from build123d import *

# Parameters (mm, degrees)
ESBO_O1_W                = 175
ESBO_O1_H                = 172.5
RESSALTO_EXTRUS_O1_DEPTH = 10
ESBO_O5_W                = 30
ESBO_O5_H                = 6
RESSALTO_EXTRUS_O5_DEPTH = 10
ESBO_O6_W                = 6
ESBO_O6_H                = 30
RESSALTO_EXTRUS_O6_DEPTH = 10
ESBO_O7_W                = 30
ESBO_O7_H                = 6
RESSALTO_EXTRUS_O7_DEPTH = 10
ESBO_O9_W                = 6.2
ESBO_O9_H                = 172.5
CORTE_EXTRUS_O2_DEPTH    = 5
ESBO_O10_R               = 1.5
CORTE_EXTRUS_O3_DEPTH    = 8
ESBO_O11_R               = 1.5
CORTE_EXTRUS_O4_DEPTH    = 8


with BuildPart() as part:
    # Esboço1 → Ressalto-extrusão1 (new body)
    with BuildSketch(Plane.XY):
        Rectangle(ESBO_O1_W, ESBO_O1_H)
    extrude(amount=RESSALTO_EXTRUS_O1_DEPTH)

    # Esboço5 → Ressalto-extrusão5 (add)
    with BuildSketch(Plane(origin=(0, 86.25, 0), x_dir=(1, 0, 0), z_dir=(0, 1, 0))):
        with Locations((-37.5, -5)):
            Rectangle(ESBO_O5_W, ESBO_O5_H)
        with Locations((37.5, -5)):
            Rectangle(ESBO_O5_W, ESBO_O5_H)
    extrude(amount=RESSALTO_EXTRUS_O5_DEPTH)

    # Esboço6 → Ressalto-extrusão6 (add)
    with BuildSketch(Plane.ZY.offset(87.5)):
        with Locations((5, 36.25)):
            Rectangle(ESBO_O6_W, ESBO_O6_H)
        with Locations((5, -36.25)):
            Rectangle(ESBO_O6_W, ESBO_O6_H)
    extrude(amount=RESSALTO_EXTRUS_O6_DEPTH)

    # Esboço7 → Ressalto-extrusão7 (add)
    with BuildSketch(Plane.XZ.offset(86.25)):
        with Locations((-37.5, 5)):
            Rectangle(ESBO_O7_W, ESBO_O7_H)
        with Locations((37.5, 5)):
            Rectangle(ESBO_O7_W, ESBO_O7_H)
    extrude(amount=RESSALTO_EXTRUS_O7_DEPTH)

    # Esboço9 → Corte-extrusão2 (cut)
    with BuildSketch(Plane.XY.offset(10)):
        with Locations((79.4, 0)):
            Rectangle(ESBO_O9_W, ESBO_O9_H)
    extrude(amount=-CORTE_EXTRUS_O2_DEPTH, mode=Mode.SUBTRACT)

    # Esboço10 → Corte-extrusão3 (cut)
    with BuildSketch(Plane.ZY.offset(87.5)):
        with Locations((5, -71.25)):
            Circle(ESBO_O10_R)
    extrude(amount=-CORTE_EXTRUS_O3_DEPTH, mode=Mode.SUBTRACT)

    # Esboço11 → Corte-extrusão4 (cut)
    with BuildSketch(Plane.XZ.offset(86.25)):
        with Locations((65, 5)):
            Circle(ESBO_O11_R)
    extrude(amount=-CORTE_EXTRUS_O4_DEPTH, mode=Mode.SUBTRACT)


solid = part.part
The model under review builds one solid part; all positions refer to its coordinate system, in mm. A direction names the side the tool comes from. Give positions to 0.01 mm unless a question says otherwise; leave off trailing zeros. Loops run counter-clockwise (first coordinate to the right, second up) from the corner with the lowest first, then second, coordinate; pieces in that order, holes last. Notation, with made-up numbers: (42, 19) -> (89, 19) arc R23 cw to (89, 41) -> close; hole circle Ø11 at (29.25, 5). An arc over 180 degrees is marked (long way). Write each question's results on one line, items separated by ' | '.
1) Tool access review of faces 1 (the face through (82.5, -1, 8)), 2 (the face through (37, 91, 8)), 3 (the face through (-92, -36, 2)), 4 (the face through (52.5, -91, 5)), 5 (the face through (-92, -51.25, 5)): name each direction out of +Z, -Z, +X, -X, +Y, -Y from which nothing blocks a thin tool from reaching the whole face with its end or side.
Conclusion:
face 1: +Z, +Y, -Y | face 2: +Z, +X, -X, +Y | face 3: -Z, -X, +Y, -Y | face 4: +Z, -Z, +X, -Y | face 5: +Z, -Z, -X, -Y
2) Take a section at A-A, the plane y = 73. Give the boundary of the cut face in (x, z), plus the area to 3 significant figures.
Conclusion:
outline: (-87.5, 0) -> (87.5, 0) -> (87.5, 10) -> (82.5, 10) -> (82.5, 5) -> (76.3, 5) -> (76.3, 10) -> (-87.5, 10) -> close | area: 1,720 mm^2
3) For line 1 along Z through (x, y) = (65, -81.5); line 2 along X through (y, z) = (-80.5, 7); line 3 along X through (y, z) = (-43.5, 7.25), list the stretches that pass through material, from the lowest coordinate up. Write a range as from..to.
Conclusion:
line 1: z = 0..3.5, 6.5..10 | line 2: x = -87.5..76.3, 82.5..87.5 | line 3: x = -97.5..76.3, 82.5..87.5
4) Draft analysis for pull direction X (two halves, no side actions). For faces 6 (the face through (-97.5, -36, 5)), 7 (the face through (-92, 21.25, 5)), 8 (the face through (22.5, -91, 5)), state which applies: pulls with the +X half, pulls with the -X half, needs draft (parallel to the pull), parting line crosses it, or undercut.
Conclusion:
face 6: pulls with the -X half | face 7: needs draft | face 8: undercut
5) Take a section at C-C, the plane x = 49. Give the boundary of the cut face in (y, z).
Conclusion:
outline: (-96.25, 2) -> (-86.25, 2) -> (-86.25, 0) -> (86.25, 0) -> (86.25, 2) -> (96.25, 2) -> (96.25, 8) -> (86.25, 8) -> (86.25, 10) -> (-86.25, 10) -> (-86.25, 8) -> (-96.25, 8) -> close
6) Insertion check: pin 1 Ø11 at (x, y) = (33.5, -92) entering from -Z; pin 2 Ø5 at (x, y) = (32.5, -89.5) entering from +Z; pin 3 Ø3 at (y, z) = (89, 4) entering from -X. Each pin has a flat end and moves straight along its axis. Give the tip position at first contact, or say it passes through.
Conclusion:
pin 1: stops at z = 2 | pin 2: stops at z = 8 | pin 3: stops at x = -52.5
7) Take a section at B-B, the plane x = -85. Give the boundary of the cut face in (y, z).
Conclusion:
outline: (-86.25, 0) -> (86.25, 0) -> (86.25, 10) -> (-86.25, 10) -> close; hole circle Ø3 at (-71.25, 5)
8) Take a section at D-D, the plane y = -36. Give the boundary of the cut face in (x, z).
Conclusion:
outline: (-97.5, 2) -> (-87.5, 2) -> (-87.5, 0) -> (87.5, 0) -> (87.5, 10) -> (82.5, 10) -> (82.5, 5) -> (76.3, 5) -> (76.3, 10) -> (-87.5, 10) -> (-87.5, 8) -> (-97.5, 8) -> close
